from build123d import *

# Parameters (mm, degrees)
F0_W     = 30
F0_H     = 65
F1_DEPTH = 5
F2_R     = 3
F4_D     = 2.5


with BuildPart() as f1:
    # F0 (on Top) → F1 (new body)
    with BuildSketch(Plane.XY):
        Rectangle(F0_W, F0_H)
    extrude(amount=F1_DEPTH)

    # F2
    f2_edges = [f1.edges().sort_by_distance(p)[0] for p in [
        (15, -32.5, 2.5),
        (15, 32.5, 2.5),
        (-15, -32.5, 2.5),
        (-15, 32.5, 2.5),
    ]]
    fillet(f2_edges, radius=F2_R)

    # F4 (through all)
    with Locations(Plane.XY.offset(5)):
        with Locations((-11.5, -29), (11.5, -29), (11.5, 29), (-11.5, 29)):
            Hole(F4_D / 2)


solid = f1.part
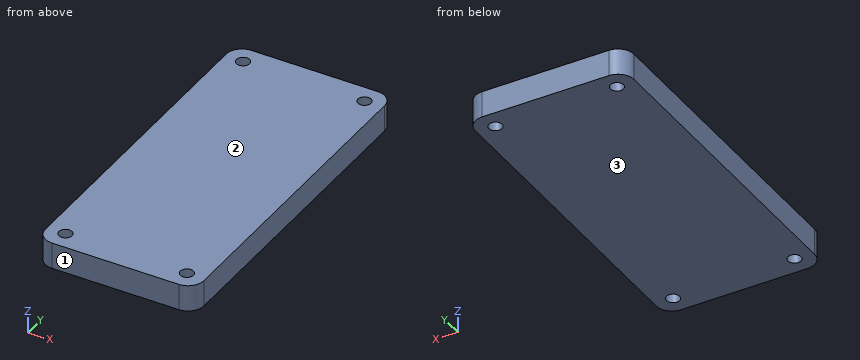
Geometry: final body of the model. Coordinates: model frame, mm. Face numbers are marked on the shaded views. Give positions to 0.01 mm unless a question says otherwise; leave off trailing zeros. Write each loop counter-clockwise with the first axis right and the second up, starting at its lowest first coordinate (ties: lowest second). Pieces come first, ordered by that corner, then holes.
(1) Ray query, line 1 (Y direction, x = 11.5, z = 2.6); line 2 (X direction, y = -30, z = 2.95). Return the intervals inside material, ascending.
(2) Mould query, pull axis Z, two halves, no side actions, for the marked faces 1, 2 and 3. Classes: released by +Z, released by -Z, zero draft, split by the parting line, or undercut.
(3) Cut plane A-A, the plane x = -11.25. Return loops of the section in (y, z).
Values follow:
1. line 1: y = -32.5 to -30.25, -27.75 to 27.75, 30.25 to 32.5
1. line 2: x = -14.96 to -12.25, -10.75 to 10.75, 12.25 to 14.96
2. face 1: zero draft
2. face 2: released by +Z
2. face 3: released by -Z
3. outline: (-32.5, 0) - (-30.22, 0) - (-30.22, 5) - (-32.5, 5) - close; (-27.78, 0) - (27.78, 0) - (27.78, 5) - (-27.78, 5) - close; (30.22, 0) - (32.5, 0) - (32.5, 5) - (30.22, 5) - close
